Part model, mm, in its own coordinate system. A direction names the side the tool comes from. Coordinates: 2 decimals unless noted, no trailing zeros. Loops run counter-clockwise (first coordinate to the right, second up) from the corner with the lowest first, then second, coordinate; pieces in that order, holes last. Notation, with made-up numbers: (-21, 1) - (-15, 1) arc R16 ccw to (-15, 13) - close; hole circle Ø7 at (67, 19). An arc over 180 degrees is marked (long way). Answer as CSV lines item,"result".
from build123d import *

# Parameters (mm, degrees)
SKETCH_1_R               = 22.5
EXTRUDE_2_DEPTH          = 5
SKETCH_5_R               = 1.5
CUT_EXTRUDE_2_DEPTH      = 11
SKETCH_6_R               = 3
CUT_EXTRUDE_3_DEPTH      = 3
SKETCH_9_R               = 1.4
EXTRUDE_5_DEPTH          = 3.5
SKETCH_10_R              = 7
EXTRUDE_6_DEPTH          = 2
CUT_EXTRUDE_4_DEPTH      = 14
CUT_EXTRUDE_4_DEPTH_BACK = 14
SKETCH_11_R              = 5


with BuildPart() as part:
    # 草图1 → 凸台-拉伸2 (new body)
    with BuildSketch(Plane(origin=(0, 0, 0), x_dir=(1, 0, 0), z_dir=(0, 1, 0))):
        with Locations(Location((0, 0, 0), (0, 0, 270))):
            Circle(SKETCH_1_R)
    extrude(amount=-EXTRUDE_2_DEPTH)

    # 草图5 → 切除-拉伸2 (cut)
    with BuildSketch(Plane(origin=(0, 0, 0), x_dir=(1, 0, 0), z_dir=(0, 1, 0))):
        with Locations(Location((0, 15, 0), (0, 0, 270))):
            Circle(SKETCH_5_R)
        with Locations(Location((15, 0, 0), (0, 0, 270))):
            Circle(SKETCH_5_R)
        with Locations(Location((0, -14.760226484, 0), (0, 0, 270))):
            Circle(SKETCH_5_R)
        with Locations(Location((-15, 0, 0), (0, 0, 270))):
            Circle(SKETCH_5_R)
    extrude(amount=-CUT_EXTRUDE_2_DEPTH, mode=Mode.SUBTRACT)

    # 草图6 → 切除-拉伸3 (cut)
    with BuildSketch(Plane(origin=(0, 0, 0), x_dir=(1, 0, 0), z_dir=(0, 1, 0))):
        with Locations(Location((0, 15, 0), (0, 0, 270))):
            Circle(SKETCH_6_R)
        with Locations(Location((15, 0, 0), (0, 0, 270))):
            Circle(SKETCH_6_R)
        with Locations(Location((0, -14.760226484, 0), (0, 0, 270))):
            Circle(SKETCH_6_R)
        with Locations(Location((-15, 0, 0), (0, 0, 270))):
            Circle(SKETCH_6_R)
    extrude(amount=-CUT_EXTRUDE_3_DEPTH, mode=Mode.SUBTRACT)

    # 草图9 → 凸台-拉伸5 (add)
    with BuildSketch(Plane(origin=(0, 0, 0), x_dir=(1, 0, 0), z_dir=(0, 1, 0))):
        with Locations(Location((0, 9.5, 0), (0, 0, 270))):
            Circle(SKETCH_9_R)
        with Locations(Location((9.5, 0, 0), (0, 0, 270))):
            Circle(SKETCH_9_R)
        with Locations(Location((0, -9.5, 0), (0, 0, 270))):
            Circle(SKETCH_9_R)
        with Locations(Location((-9.5, 0, 0), (0, 0, 270))):
            Circle(SKETCH_9_R)
    extrude(amount=EXTRUDE_5_DEPTH)

    # 草图10 → 凸台-拉伸6 (add)
    with BuildSketch(Plane(origin=(0, 0, 0), x_dir=(1, 0, 0), z_dir=(0, 1, 0))):
        with Locations(Location((0, 0, 0), (0, 0, 270))):
            Circle(SKETCH_10_R)
    extrude(amount=EXTRUDE_6_DEPTH)

    # 草图11 → 切除-拉伸4 (cut, two sides: drawn at the far end of the back side and taken through both)
    with BuildSketch(Plane(origin=(0, 0, 0), x_dir=(1, 0, 0), z_dir=(0, 1, 0)).offset(-CUT_EXTRUDE_4_DEPTH_BACK)):
        with Locations(Location((0, 0, 0), (0, 0, 270))):
            Circle(SKETCH_11_R)
    extrude(amount=CUT_EXTRUDE_4_DEPTH + CUT_EXTRUDE_4_DEPTH_BACK, mode=Mode.SUBTRACT)


solid = part.part
Q1. Saw through at A-A (x = 15). Give the cut face in (y, z), then the cut area to 3 significant figures.
Results:
outline,"(-5, -16.77) - (0, -16.77) - (0, -3) - (-3, -3) - (-3, -1.5) - (-5, -1.5) - close; (-5, 1.5) - (-3, 1.5) - (-3, 3) - (0, 3) - (0, 16.77) - (-5, 16.77) - close"
area,"144 mm^2"
Q2. Saw through at D-D (z = 0). Count the separate pieces of the cut face and the enclosed holes in it, then the cut area to 3 significant figures.
Results:
separate pieces,"4"
enclosed holes,"0"
area,"155 mm^2"
Q3. Two-plate mould, pull along Z, no slides. Class faces 3 (the face through (-8.618, -2.465, 20.784)), 4 (the face through (0.06, 1.73, 8.1)), 5 (the face through (0, 3.5, 9)): released by +Z, released by -Z, zero draft, split by the parting line, or undercut.
Results:
face 3,"split by the parting line"
face 4,"undercut"
face 5,"zero draft"
Q4. Saw through at B-B (y = -4). Give the cut face in (x, z), then the cut area to 3 significant figures.
Results:
outline,"circle Ø45 at (0, 0); hole circle Ø3 at (-15, 0); hole circle Ø10 at (0, 0); hole circle Ø3 at (0, -15); hole circle Ø3 at (0, 14.76); hole circle Ø3 at (15, 0)"
area,"1,480 mm^2"
Q5. Saw through at C-C (z = -15). Give the cut face in (x, y), then the cut area to 3 significant figures.
Results:
outline,"(-16.77, -5) - (-1.5, -5) - (-1.5, -3) - (-3, -3) - (-3, 0) - (-16.77, 0) - close; (1.5, -5) - (16.77, -5) - (16.77, 0) - (3, 0) - (3, -3) - (1.5, -3) - close"
area,"144 mm^2"
Q6. Which spindle directions (+Z, -Z, +X, -X, +Y, -Y) get a long thin tool onto all of the face, cutting with end or side? Do faces 1 (the face through (12.07, -1.48, -0.65)), 2 (the face through (0, 3.5, -10)). Say none if no direction does.
Results:
face 1,"+Y"
face 2,"+Z, -Z, +X, -X, +Y"
Q7. Wall check: L1, parallel to X at y = -2.3, z = 0; L2, parallel to X at y = -4.1, z = 0; L3, parallel to Z at x = -4, y = -2.75. Give the ranges that are in metal, low to high.
Results:
L1,"x = -22.5 to -18, -12 to -5, 5 to 12, 18 to 22.5"
L2,"x = -22.5 to -16.5, -13.5 to -5, 5 to 13.5, 16.5 to 22.5"
L3,"z = -22.14 to -3, 3 to 22.14"
Q8. Flat gauge pins, fed straight in: pin 1 (1.8 mm diameter, centred on x = -1, z = 15, fed in from +Y); pin 2 (5 mm diameter, centred on x = -15, z = 0, fed in from -Y); pin 3 (11 mm diameter, centred on x = -1, z = 2, fed in from +Y); pin 4 (1 mm diameter, centred on y = -3.5, z = 0, fed in from -X). Where does each tip first touch, or does it go through?
Results:
pin 1,"stops at y = -3"
pin 2,"stops at y = -5"
pin 3,"stops at y = 2"
pin 4,"stops at x = -22.5"
